Autodesk Inventor part; units mm, degrees
ref_plane "РабПлоскость1" through (-8.75, 20, 95.5) normal (-0.9659258, 0.258819, 0) x (0, 0, -1)
ref_plane "YZ Plane" through (0, 0, 0) normal (1, 0, 0) x (0, 1, 0)
ref_plane "XZ Plane" through (0, 0, 0) normal (0, 1, 0) x (-1, 0, 0)
sketch "Эскиз1" plane through (0, 0, 0) normal (0, 1, 0) x (-1, 0, 0)
  line L0 (8.75, 95.5) -> (-8.75, 95.5)
  line L1 (-8.75, 95.5) -> (-8.75, -95.5)
  line L2 (-8.75, -95.5) -> (8.75, -95.5)
  line L3 (8.75, -95.5) -> (8.75, 95.5)
  line L4 (8.75, -95.5) -> (-8.75, 95.5) construction
  line L5 (-8.75, -95.5) -> (8.75, 95.5) construction
  point P0 (0, 0)
  point P1 (0, 0)
  dimension "d0" = 17.5
  dimension "d1" = 191
extrude "Выдавливание1" add sketch "Эскиз1" along normal blind 75
sketch "Эскиз2" plane through (-8.75, 0, -95.5) normal (-1, 0, 0) x (0, 0, 1)
  line L0 (191, 0) -> (191, 75) construction
  line L1 (191, 20) -> (0, 20)
  line L2 (0, 0) -> (0, 75) construction
  line L3 (0, 0) -> (191, 0) construction
  point P0 (95.5, 0)
  dimension "d4" = 20
ref_plane "РабПлоскость1" through (-8.75, 20, 95.5) normal (-0.9659258, 0.258819, 0) x (0, 0, -1)
split "Разделение1" plane through (-8.75, 20, 95.5) removes the side toward (-0.9659258, 0.258819, 0)
sketch "Эскиз3" plane through (5.9872, 75, -95.5) normal (-0.9659258, 0.258819, 0) x (0, 0, 1)
  line L0 (0, -56.9402) -> (0, 0) construction
  line L1 (0, 0) -> (191, 0) construction
  line L2 (191, 0) -> (191, -56.9402) construction
  line L3 (191, -56.9402) -> (0, -56.9402) construction
  line L4 (191, -71.7294) -> (191, 0.7151) construction
  line L5 (191, -53.9402) -> (0, -30.4883) construction
  line L6 (0, -71.7294) -> (0, 0.7151) construction
  line L7 (17.5, -22.562) -> (43, -25.693)
  line L8 (43, -25.693) -> (43, -8.5653)
  line L9 (43, -8.5653) -> (17.5, -5.4343)
  line L10 (17.5, -5.4343) -> (17.5, -22.562)
  line L11 (47, 0) -> (47, -56.9402) construction
  line L12 (191, -56.9402) -> (0, -56.9402) construction
  line L13 (94, 0) -> (94, -56.9402) construction
  line L14 (142, 0) -> (142, -56.9402) construction
  line L15 (43, -8.5653) -> (47, -8.5653) construction
  line L16 (60.5, -27.8417) -> (60.5, -9.2028)
  line L17 (60.5, -9.2028) -> (90, -12.8249)
  line L18 (90, -12.8249) -> (90, -31.4639)
  line L19 (90, -31.4639) -> (60.5, -27.8417)
  line L20 (90, -12.8249) -> (94, -12.8249) construction
  line L21 (105, -33.3056) -> (105, -13.6592)
  line L22 (105, -13.6592) -> (138, -17.7111)
  line L23 (138, -17.7111) -> (138, -37.3575)
  line L24 (138, -37.3575) -> (105, -33.3056)
  line L25 (138, -17.7111) -> (142, -17.7111) construction
  line L26 (149.5, -17.1081) -> (149.5, -38.7695)
  line L27 (149.5, -38.7695) -> (187, -43.374)
  line L28 (187, -43.374) -> (187, -21.7125)
  line L29 (187, -21.7125) -> (149.5, -17.1081)
  line L30 (187, -21.7125) -> (191, -21.7125) construction
  point P0 (95.5, -73.994)
  dimension "d6" = 3
  dimension "d7" = 7
  dimension "d8" = 10
  dimension "d9" = 25.5
  dimension "d10" = 27
  dimension "d11" = 4
  dimension "d12" = 29.5
  dimension "d13" = 28.5
  dimension "d14" = 33
  dimension "d15" = 29.5
  dimension "d16" = 37.5
  dimension "d17" = 31.5
  dimension "d36" = 49
  dimension "d37" = 48
  dimension "d38" = 47
extrude "Выдавливание2" cut sketch "Эскиз3" against normal through all
sketch "Эскиз5" plane through (0, 0, 0) normal (0, 1, 0) x (-1, 0, 0)
  line L0 (8.75, -95.5) -> (-8.75, -95.5) construction
  line L1 (-8.75, -95.5) -> (-8.75, 95.5) construction
  line L2 (-8.75, 95.5) -> (8.75, 95.5) construction
  line L3 (8.75, 95.5) -> (8.75, -95.5)
  line L4 (8.75, -95.5) -> (18.75, -95.5)
  line L5 (18.75, -95.5) -> (18.75, 85.5)
  line L6 (18.75, 95.5) -> (8.75, 95.5)
  line L7 (8.75, 95.5) -> (8.75, -95.5) construction
  line L8 (18.75, 85.5) -> (18.75, 95.5)
  line L9 (24.25, 0) -> (-14.25, 0) construction
  point P0 (0, 0)
  point P1 (8.75, 95.5)
  dimension "d26" = 10
extrude "Выдавливание5" add sketch "Эскиз5" along normal blind 2
sketch "Эскиз4" plane through (5.9872, 75, -95.5) normal (-0.9659258, 0.258819, 0) x (0, 0, 1)
  line L0 (191, 0.7151) -> (0, 0.7151) construction
  line L1 (95.5, 0.7151) -> (95.5, -56.9402) construction
  line L2 (191, -56.9402) -> (0, -56.9402) construction
  line L3 (191, -71.7294) -> (191, 0.7151) construction
  line L4 (0, -71.7294) -> (0, 0.7151) construction
  line L5 (191, -28.1126) -> (0, -28.1126) construction
  line L6 (191, -76.2587) -> (191, -56.9402) construction
  circle A0 centre (5, -51.9402) radius 0.5
  circle A1 centre (5, -4.2849) radius 0.5
  line L7 (0, -56.9402) -> (0, 0)
  line L8 (0, -56.9402) -> (10, -56.9402)
  line L9 (10, -56.9402) -> (10, -46.9402)
  line L10 (10, -46.9402) -> (0, -46.9402)
  line L11 (0, -46.9402) -> (0, -56.9402)
  line L12 (10, -56.9402) -> (0, -46.9402) construction
  line L13 (0, -56.9402) -> (10, -46.9402) construction
  circle A2 centre (186, -4.2849) radius 0.5
  point P0 (95.5, -73.994)
  point P1 (95.5, -28.1126)
  dimension "d46" = 10
  dimension "d47" = 1
hole "Отверстие1" at (-7.4559, 24.8296, -90.5) at (4.8782, 70.8611, -90.5) at (4.8782, 70.8611, 90.5) direction (0.9659258, -0.258819, 0) diameter 1 depth 2.5 tip angle 118 countersink diameter 1.5 countersink angle 90
sketch "Эскиз6" plane through (0, 2, 0) normal (0, 1, 0) x (1, 0, 0)
  line L0 (-8.75, -95.5) -> (-8.75, 95.5) construction
  line L1 (-18.75, 95.5) -> (-8.75, 95.5) construction
  line L2 (-18.75, -95.5) -> (-18.75, 95.5) construction
  line L3 (-8.75, -95.5) -> (-18.75, -95.5) construction
  line L4 (8.75, -95.5) -> (-8.75, -95.5) construction
  line L5 (8.75, 95.5) -> (8.75, -95.5) construction
  line L6 (-8.75, 95.5) -> (8.75, 95.5) construction
  line L7 (-8.75, -95.5) -> (-18.75, -95.5) construction
  line L8 (-18.75, -95.5) -> (-18.75, -85.5) construction
  line L9 (-18.75, -85.5) -> (-8.75, -85.5) construction
  line L10 (-8.75, -85.5) -> (-8.75, -95.5) construction
  circle A0 centre (-13.75, -85.5) radius 0.5
  circle A1 centre (-13.75, -36.5) radius 0.5
  circle A2 centre (-13.75, 11.5) radius 0.5
  circle A3 centre (-13.75, 58.5) radius 0.5
  point P0 (0, 0)
  dimension "d50" = 1
  dimension "d51" = 49
  dimension "d52" = 48
  dimension "d53" = 47
hole "Отверстие2" at (-13.75, 2, -58.5) at (-13.75, 2, -11.5) at (-13.75, 2, 36.5) at (-13.75, 2, 85.5) direction (0, -1, 0) diameter 1 end through all countersink diameter 1.5 countersink angle 90
properties part number "SortBoard-Frame"
Can you work these out from the model? Positions are in its coordinate system, mm. A direction names the side the tool comes from. Coordinates: 2 decimals unless noted, no trailing zeros. Order: outer loops, then holes, each group sorted by start corner. A loop starts at its lowest first (then second) coordinate and runs counter-clockwise, first axis right, second up. Notation, with made-up numbers: (-12, -39) - (3, -39) arc R27 cw to (3, -23) - close; hole circle Ø7 at (28, -25.75). An arc over 180 degrees is marked (long way). Answer as a JSON object with one key per item and string values. Group by question number.
Q1. Imagine slicing it at C-C (y = 14.5). Please give me the cut outline in (x, z), and give its area (3 significant figures).
Q2. Imagine slicing it at A-A (z = -18). Please give me the cut outline in (x, y), and give its area (3 significant figures).
Q3. Imagine slicing it at D-D (z = 31). Please give me the cut outline in (x, y).
Q4. On a 3-axis mill with a long thin cutter (end or side, diameter ignored), from which of +Z, -Z, +X, -X, +Y, -Y can I reach the whole of each face in a straight line? I mean faces 1 (the face through (-8.75, 11, -1)), 2 (the face through (6.62, 67.56, -65.07)), 3 (the face through (8.75, 37, 1)), 4 (the face through (3.683, 44.892, -20.044)), 5 (the face through (1, 29, 95.5)). Say none if no direction works.
Q5. I need wall thicknesses on line 1 (Z direction, x = -13.75, y = 0.95); line 2 (X direction, y = 0.85, z = -58.5); line 3 (X direction, y = 11, z = 77). Which ranges of each line are inside material? Lowest first, please. Write a range as from..to.
Q6. Will these pins go through, and if not, where does the flat tip stop? P1, Ø1, axis at y = 59.5, z = 49, coming from the -X side; P2, Ø9, axis at y = 11, z = -25.5, coming from the -X side; P3, Ø8, axis at x = -14, z = -45.5, coming from the +Y side.
Q7. We'd pull the mould along Y, two halves only. Please class faces 6 (the face through (3, 42, 91.5)), 7 (the face through (-1.485, 47.115, 1.337)), 8 (the face through (1, 29, -95.5)): +Y half, -Y half, draft (parallel to the pull), parting line (faces both ways), or undercut.
Q8. Imagine slicing it at B-B (z = -39.5). Please give me the cut outline in (x, y).
Determined:
{
 "1": {"outline": "(-8.75, -95.5) - (8.75, -95.5) - (8.75, 95.5) - (-8.75, 95.5) - close", "area": "3,340 mm2"},
 "2": {"outline": "(-18.75, 0) - (8.75, 0) - (8.75, 43.27) - (-1.76, 46.09) - (-8.75, 20) - (-8.75, 2) - (-18.75, 2) - close; (3.07, 64.09) - (8.75, 62.57) - (8.75, 75) - (5.99, 75) - close", "area": "771 mm2"},
 "3": {"outline": "(-18.75, 0) - (8.75, 0) - (8.75, 37.05) - (-3.32, 40.28) - (-8.75, 20) - (-8.75, 2) - (-18.75, 2) - close; (1.77, 59.26) - (8.75, 57.39) - (8.75, 75) - (5.99, 75) - close"},
 "4": {"face 1": "+Z, -Z, -X, +Y", "face 2": "-X", "face 3": "+Z, -Z, +X, +Y, -Y", "face 4": "+X", "face 5": "+Z, +X, -X, +Y, -Y"},
 "5": {"line 1": "z = -95.5..-59, -58..-12, -11..36, 37..85, 86..95.5", "line 2": "x = -18.75..-14.25, -13.25..8.75", "line 3": "x = -8.75..8.75"},
 "6": {"P1": "stops at x = 1.7", "P2": "stops at x = -8.75", "P3": "stops at y = 2"},
 "7": {"face 6": "undercut", "face 7": "+Y half", "face 8": "draft"},
 "8": {"outline": "(-18.75, 0) - (8.75, 0) - (8.75, 75) - (5.99, 75) - (-8.75, 20) - (-8.75, 2) - (-18.75, 2) - close"}
}
